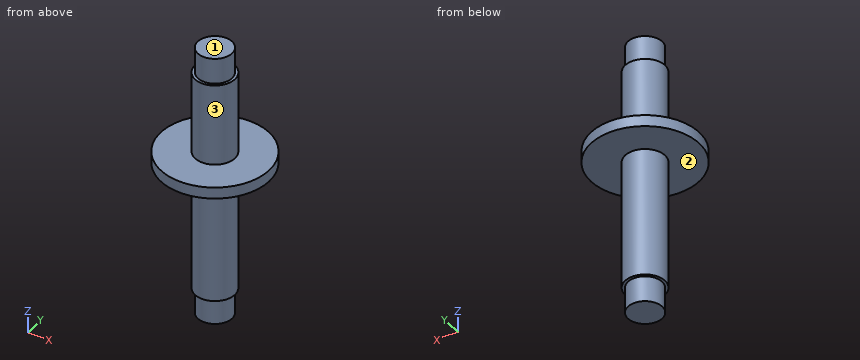
```python
from build123d import *

# Parameters (mm, degrees)
CROQUIS1_R              = 3
SALIENTE_EXTRUIR1_DEPTH = 4.5
CROQUIS2_R              = 3.5
SALIENTE_EXTRUIR2_DEPTH = 22.75
CROQUIS3_R              = 9.5
SALIENTE_EXTRUIR3_DEPTH = 2
CROQUIS4_R              = 3.5
SALIENTE_EXTRUIR4_DEPTH = 14.35
CROQUIS5_R              = 3
SALIENTE_EXTRUIR5_DEPTH = 4.5


with BuildPart() as part:
    # Croquis1 → Saliente-Extruir1 (new body)
    with BuildSketch(Plane.XY):
        Circle(CROQUIS1_R)
    extrude(amount=SALIENTE_EXTRUIR1_DEPTH)

    # Croquis2 → Saliente-Extruir2 (add)
    with BuildSketch(Plane.XY.offset(4.5)):
        Circle(CROQUIS2_R)
    extrude(amount=SALIENTE_EXTRUIR2_DEPTH)

    # Croquis3 → Saliente-Extruir3 (add)
    with BuildSketch(Plane.XY.offset(27.25)):
        Circle(CROQUIS3_R)
    extrude(amount=SALIENTE_EXTRUIR3_DEPTH)

    # Croquis4 → Saliente-Extruir4 (add)
    with BuildSketch(Plane.XY.offset(29.25)):
        Circle(CROQUIS4_R)
    extrude(amount=SALIENTE_EXTRUIR4_DEPTH)

    # Croquis5 → Saliente-Extruir5 (add)
    with BuildSketch(Plane.XY.offset(43.6)):
        Circle(CROQUIS5_R)
    extrude(amount=SALIENTE_EXTRUIR5_DEPTH)


solid = part.part
```
Geometry check sheet. Reference: the model listing, model coordinates, mm. Face numbers are marked on the shaded views. A direction names the side the tool comes from. Round coordinates to 2 decimals unless told otherwise and drop trailing zeros. Loops run counter-clockwise (first coordinate to the right, second up) from the corner with the lowest first, then second, coordinate; pieces in that order, holes last. Notation, with made-up numbers: (-19.75, 55.25) - (-14.75, 55.25) arc R7 cw to (-14.75, 64.25) - close; hole circle Ø4 at (68.5, 19). An arc over 180 degrees is marked (long way). Write each question's results on one line, items separated by ' | '. Start each with the question number.
Q1. Thickness scan on line 1 (Z direction, x = -8.5, y = 0.25); line 2 (Z direction, x = 2.75, y = 2); line 3 (X direction, y = 0.25, z = 5). Record the ranges inside material, lowest first. Write a range as [from, to].
Q2. Cross-section at A-A on x = 0. Enter the section's corners in (y, z), and give its area (3 significant figures).
Q3. Cross-section at D-D on z = 39. Enter the section's corners in (x, y), and give its area (3 significant figures).
Q4. Gauge pin test, flat ends, axial feed: P1, Ø8, axis at x = -4, z = 8.5, coming from the -Y side; P2, Ø3, axis at x = 6.5, z = 30, coming from the +Y side; P3, Ø3, axis at x = -6.5, z = 29.5, coming from the -Y side; P4, Ø1.5, axis at x = 4.5, z = 13.5, coming from the +Y side. Record the tip position at first contact, or that the pin passes through.
Q5. Cross-section at B-B on y = -1.5. Enter the section's corners in (x, z), and give its area (3 significant figures).
Q6. Cross-section at C-C on z = 4. Enter the section's corners in (x, y), and give its area (3 significant figures).
Q7. Access from +Z, -Z, +X, -X, +Y, -Y to the whole of each face (thin tool, end or side, straight path). Record for the marked faces 1, 2 and 3.
Answers below:
1) line 1: z = [27.25, 29.25] | line 2: z = [4.5, 43.6] | line 3: x = [-3.49, 3.49]
2) outline: (-9.5, 27.25) - (-3.5, 27.25) - (-3.5, 4.5) - (-3, 4.5) - (-3, 0) - (3, 0) - (3, 4.5) - (3.5, 4.5) - (3.5, 27.25) - (9.5, 27.25) - (9.5, 29.25) - (3.5, 29.25) - (3.5, 43.6) - (3, 43.6) - (3, 48.1) - (-3, 48.1) - (-3, 43.6) - (-3.5, 43.6) - (-3.5, 29.25) - (-9.5, 29.25) - close | area: 352 mm²
3) outline: circle Ø7 at (0, 0) | area: 38.5 mm²
4) P1: stops at y = -3.5 | P2: stops at y = 7.95 | P3: stops at y = -8.06 | P4: passes through
5) outline: (-9.38, 27.25) - (-3.16, 27.25) - (-3.16, 4.5) - (-2.6, 4.5) - (-2.6, 0) - (2.6, 0) - (2.6, 4.5) - (3.16, 4.5) - (3.16, 27.25) - (9.38, 27.25) - (9.38, 29.25) - (3.16, 29.25) - (3.16, 43.6) - (2.6, 43.6) - (2.6, 48.1) - (-2.6, 48.1) - (-2.6, 43.6) - (-3.16, 43.6) - (-3.16, 29.25) - (-9.38, 29.25) - close | area: 319 mm²
6) outline: circle Ø6 at (0, 0) | area: 28.3 mm²
7) face 1: +Z, +X, -X, +Y, -Y | face 2: -Z | face 3: +Z
